Could you check a few things on this model? Use its own coordinates, in mm. A direction names the side the tool comes from. Give positions to 0.01 mm unless a question says otherwise; leave off trailing zeros. Write each loop counter-clockwise with the first axis right and the second up, starting at its lowest first coordinate (ties: lowest second). Pieces come first, ordered by that corner, then holes. Notation, with made-up numbers: (48.25, 35.5) - (66.25, 35.5) arc R29 ccw to (66.25, 69.5) - close; hole circle Ø3 at (-21, 9). An arc over 180 degrees is marked (long way). Write item = value, one per line.
from build123d import *

# Parameters (mm, degrees)
BOSS_EXTRUDE1_DEPTH = 10
CUT_EXTRUDE1_REACH  = 151.3
FILLET1_R           = 1
FILLET2_R           = 1


with BuildPart() as part:
    # Sketch2 → Boss-Extrude1 (new body)
    with BuildSketch(Plane.XY):
        with BuildLine():
            Line((0, -1), (60, -1))
            Line((60, -1), (80, -1))
            ThreePointArc((80, -1), (81, 0), (80, 1))
            Line((80, 1), (60.649049017, 1))
            Line((60.649049017, 1), (5.5, 124.698801533))
            Line((5.5, 124.698801533), (5.5, 1))
            Line((5.5, 1), (0, 1))
            Line((0, 1), (-2, 1))
            Line((-2, 1), (-7.5, 1))
            Line((-7.5, 1), (-7.5, 124.698801533))
            Line((-7.5, 124.698801533), (-62.649049017, 1))
            Line((-62.649049017, 1), (-82, 1))
            ThreePointArc((-82, 1), (-83, 0), (-82, -1))
            Line((-82, -1), (-62, -1))
            Line((-62, -1), (-2, -1))
            Line((-2, -1), (0, -1))
        make_face()
        Polygon((7.59488235, 1), (58.459284316, 1), (33.027083333, 58.044189121), align=None, mode=Mode.SUBTRACT)
        Polygon((31.932200983, 60.5), (7.5, 5.698801533), (7.5, 115.301198467), align=None, mode=Mode.SUBTRACT)
        Polygon((-35.027083333, 58.044189121), (-9.59488235, 1), (-60.459284316, 1), align=None, mode=Mode.SUBTRACT)
        Polygon((-9.5, 115.301198467), (-33.932200983, 60.5), (-9.5, 5.698801533), align=None, mode=Mode.SUBTRACT)
    extrude(amount=BOSS_EXTRUDE1_DEPTH)

    # Sketch3 → Cut-Extrude1 (cut, up to next)
    with BuildSketch(Plane(origin=(0, 1, 0), x_dir=(1, 0, 0), z_dir=(0, 1, 0)), mode=Mode.PRIVATE) as cut_extrude1_sk1:
        with BuildLine():
            Line((-72.324524509, -3.585786438), (-73.03163129, -4.292893219))
            ThreePointArc((-73.03163129, -4.292893219), (-73.324524509, -5), (-73.03163129, -5.707106781))
            Line((-73.03163129, -5.707106781), (-72.324524509, -6.414213562))
            Line((-72.324524509, -6.414213562), (-71.617417727, -5.707106781))
            ThreePointArc((-71.617417727, -5.707106781), (-71.324524509, -5), (-71.617417727, -4.292893219))
            Line((-71.617417727, -4.292893219), (-72.324524509, -3.585786438))
        make_face()
    cut_extrude1_tool1 = extrude(cut_extrude1_sk1.sketch, amount=-CUT_EXTRUDE1_REACH, mode=Mode.PRIVATE) & part.part
    # Sketch3 → Cut-Extrude1 (cut, up to next)
    with BuildSketch(Plane(origin=(0, 1, 0), x_dir=(1, 0, 0), z_dir=(0, 1, 0)), mode=Mode.PRIVATE) as cut_extrude1_sk2:
        with BuildLine():
            Line((69.617417727, -5.707106781), (70.324524509, -6.414213562))
            Line((70.324524509, -6.414213562), (71.03163129, -5.707106781))
            ThreePointArc((71.03163129, -5.707106781), (71.324524509, -5), (71.03163129, -4.292893219))
            Line((71.03163129, -4.292893219), (70.324524509, -3.585786438))
            Line((70.324524509, -3.585786438), (69.617417727, -4.292893219))
            ThreePointArc((69.617417727, -4.292893219), (69.324524509, -5), (69.617417727, -5.707106781))
        make_face()
    cut_extrude1_tool2 = extrude(cut_extrude1_sk2.sketch, amount=-CUT_EXTRUDE1_REACH, mode=Mode.PRIVATE) & part.part
    add(cut_extrude1_tool1.solids().sort_by_distance((-72.324525, 1, 5))[0], mode=Mode.SUBTRACT)
    add(cut_extrude1_tool2.solids().sort_by_distance((70.324525, 1, 5))[0], mode=Mode.SUBTRACT)

    # Fillet1
    fillet1_edges = [part.edges().sort_by_distance(p)[0] for p in [
        (5.5, 124.698801533, 5),
    ]]
    fillet(fillet1_edges, radius=FILLET1_R)

    # Fillet2
    fillet2_edges = [part.edges().sort_by_distance(p)[0] for p in [
        (-7.5, 124.698801533, 5),
    ]]
    fillet(fillet2_edges, radius=FILLET2_R)


solid = part.part
1. I need wall thicknesses on line 1 (X direction, y = 95, z = 6); line 2 (X direction, y = 86, z = 5.5); line 3 (X direction, y = 37, z = 3.25). Which ranges of each line are inside material? Lowest first, please.
Filled sheet:
line_1 = -20.74 to -18.55, -9.5 to -7.5, 5.5 to 7.5, 16.55 to 18.74
line_2 = -24.75 to -22.56, -9.5 to -7.5, 5.5 to 7.5, 20.56 to 22.75
line_3 = -46.6 to -44.41, -25.64 to -23.46, -9.5 to -7.5, 5.5 to 7.5, 21.46 to 23.64, 42.41 to 44.6
2. If we section it at C-C, the plane y = 9: Please give me the cut outline in (x, z), and give its area (3 significant figures).
Filled sheet:
outline = (-59.08, 0) - (-56.89, 0) - (-56.89, 10) - (-59.08, 10) - close; (-13.16, 0) - (-10.97, 0) - (-10.97, 10) - (-13.16, 10) - close; (-9.5, 0) - (-7.5, 0) - (-7.5, 10) - (-9.5, 10) - close; (5.5, 0) - (7.5, 0) - (7.5, 10) - (5.5, 10) - close; (8.97, 0) - (11.16, 0) - (11.16, 10) - (8.97, 10) - close; (54.89, 0) - (57.08, 0) - (57.08, 10) - (54.89, 10) - close
area = 128 mm2
3. If we section it at A-A, the plane z = 8: Please give me the cut outline in (x, y).
Filled sheet:
outline = (-82, -1) - (80, -1) arc R1 ccw to (80, 1) - (60.65, 1) - (7.41, 120.41) arc R1 ccw to (5.5, 120) - (5.5, 1) - (-7.5, 1) - (-7.5, 120) arc R1 ccw to (-9.41, 120.41) - (-62.65, 1) - (-82, 1) arc R1 ccw to start; hole (-60.46, 1) - (-9.59, 1) - (-35.03, 58.04) - close; hole (-33.93, 60.5) - (-9.5, 5.7) - (-9.5, 115.3) - close; hole (7.5, 5.7) - (31.93, 60.5) - (7.5, 115.3) - close; hole (7.59, 1) - (58.46, 1) - (33.03, 58.04) - close
4. Thinking about a two-plate mould opening in X: for faces 5 (the face through (20.49, 29.92, 4.93)), 6 (the face through (-25.7, 37.7, 0)), 7 (the face through (34.404, 59.868, 4.93)), which applies, pulls with the +X half, pulls with the -X half, needs draft (parallel to the pull), parting line crosses it, or undercut?
Filled sheet:
face_5 = undercut
face_6 = needs draft
face_7 = pulls with the +X half
5. If we section it at D-D, the plane y = 85: Please give me the cut outline in (x, z), and give its area (3 significant figures).
Filled sheet:
outline = (-25.2, 0) - (-23.01, 0) - (-23.01, 10) - (-25.2, 10) - close; (-9.5, 0) - (-7.5, 0) - (-7.5, 10) - (-9.5, 10) - close; (5.5, 0) - (7.5, 0) - (7.5, 10) - (5.5, 10) - close; (21.01, 0) - (23.2, 0) - (23.2, 10) - (21.01, 10) - close
area = 83.8 mm2
6. Which directions (+Z, -Z, +X, -X, +Y, -Y) give clear straight access to the entire face, cutting with the end or side of a thin tool? Please do faces 1 (the face through (73, 1, 5)), 2 (the face through (-21.887, 33.483, 4.93)), 3 (the face through (-70, 1, 5)), 4 (the face through (-1, 1, 5)).
Filled sheet:
face_1 = +Z, -Z, +X, +Y
face_2 = +Z, -Z
face_3 = +Z, -Z, -X, +Y
face_4 = +Z, -Z, +Y
7. For pin 1 (3 mm diameter, centred on y = 80.5, z = 4.5, fed in from -X); pin 2 (10 mm diameter, centred on x = 35.5, y = 81, fed in from -Z); pin 3 (5 mm diameter, centred on y = 38, z = 8.5, fed in from +X); pin 4 (5 mm diameter, centred on x = -1.5, z = 3, fed in from +Y), each with a flat end and sliding along its axis, tell me the tip position at first contact or that it passes through.
Filled sheet:
pin_1 = -27.87
pin_2 = through
pin_3 = 45.27
pin_4 = 1
8. If we section it at B-B, the plane x = 26.5: Please give me the cut outline in (y, z), and give its area (3 significant figures).
Filled sheet:
outline = (-1, 0) - (1, 0) - (1, 10) - (-1, 10) - close; (43.4, 0) - (48.32, 0) - (48.32, 10) - (43.4, 10) - close; (72.68, 0) - (77.6, 0) - (77.6, 10) - (72.68, 10) - close
area = 118 mm2
